```python
from build123d import *

# Parameters (mm, degrees)
SKETCH1_W           = 448
SKETCH1_H           = 131.3
BOSS_EXTRUDE1_DEPTH = 510
SKETCH2_W           = 482
SKETCH2_H           = 131.3
BOSS_EXTRUDE2_DEPTH = 5
CUT_EXTRUDE1_DEPTH  = 511


with BuildPart() as part:
    # Sketch1 → Boss-Extrude1 (new body)
    with BuildSketch(Plane.XY):
        Rectangle(SKETCH1_W, SKETCH1_H)
    extrude(amount=BOSS_EXTRUDE1_DEPTH)

    # Sketch2 → Boss-Extrude2 (add)
    with BuildSketch(Plane(origin=(0, 0, 0), x_dir=(-1, 0, 0), z_dir=(0, 0, -1))):
        Rectangle(SKETCH2_W, SKETCH2_H)
    extrude(amount=-BOSS_EXTRUDE2_DEPTH)

    # Sketch3 → Cut-Extrude1 (cut, through all)
    with BuildSketch(Plane(origin=(0, 0, 0), x_dir=(-1, 0, 0), z_dir=(0, 0, -1))):
        with BuildLine():
            Line((-234.4, 31.975), (-230.6, 31.975))
            ThreePointArc((-230.6, 31.975), (-227.2, 28.575), (-230.6, 25.175))
            Line((-230.6, 25.175), (-234.4, 25.175))
            ThreePointArc((-234.4, 25.175), (-237.8, 28.575), (-234.4, 31.975))
        make_face()
        with BuildLine():
            Line((234.4, 25.175), (230.6, 25.175))
            ThreePointArc((230.6, 25.175), (227.2, 28.575), (230.6, 31.975))
            Line((230.6, 31.975), (234.4, 31.975))
            ThreePointArc((234.4, 31.975), (237.8, 28.575), (234.4, 25.175))
        make_face()
    cut_extrude1 = extrude(amount=-CUT_EXTRUDE1_DEPTH, mode=Mode.SUBTRACT)

    # Mirror1: Cut-Extrude1 across plane
    add(cut_extrude1.mirror(Plane.ZX), mode=Mode.SUBTRACT)


solid = part.part
```
Could you check a few things on this model? Use its own coordinates, in mm. A direction names the side the tool comes from. Give positions to 0.01 mm unless a question says otherwise; leave off trailing zeros. Order: outer loops, then holes, each group sorted by start corner. A loop starts at its lowest first (then second) coordinate and runs counter-clockwise, first axis right, second up.
Q1. I'm going to push flat-ended pins straight in: P1, Ø5, axis at y = 10.5, z = 220.5, coming from the +X side; P2, Ø18.5, axis at x = -236, y = -4, coming from the +Z side; P3, Ø1, axis at y = 11, z = 86, coming from the -X side. Where does each tip first touch, or does it pass through?
Q2. Suppose I cut it at A-A, the plane y = -52. Write out the boundary of the cut face in (x, z), and give its area (3 significant figures).
Q3. For faces 1 (the flat face through (233, 1, 5)), 2 (the flat face through (-232, 1, 5)), 3 (the flat face through (-3, 1, 510)), which set-ups out of +Z, -Z, +X, -X, +Y, -Y let a thin tool reach every point of the face, with its end or its side?
Q4. Suppose I cut it at B-B, the plane z = 183. Write out the boundary of the cut face in (x, y).
Q5. If I drill on line 1 along X through (y, z) = (-14.5, 54), over which ranges is the centre line in solid material (lowest first)?
Solution:
1. P1: stops at x = 224
1. P2: stops at z = 5
1. P3: stops at x = -224
2. outline: (-241, 0) - (241, 0) - (241, 5) - (224, 5) - (224, 510) - (-224, 510) - (-224, 5) - (-241, 5) - close
2. area: 229,000 mm2
3. face 1: +Z, +X, +Y, -Y
3. face 2: +Z, -X, +Y, -Y
3. face 3: +Z, +X, -X, +Y, -Y
4. outline: (-224, -65.65) - (224, -65.65) - (224, 65.65) - (-224, 65.65) - close
5. line 1: x = -224 to 224
